from build123d import *

# Parameters (mm, degrees)
F2_ANGLE_BACK   = 15
F2_ANGLE        = 30
F2_COPIES_COUNT = 7


# Not quite as in the source:
# - a pattern or mirror of a feature is missing from the dataset's text; its kind, count and spacing are read off the source's solid


with BuildPart() as f1:
    # F0 (on Right) → F1 (revolve)
    with BuildSketch(Plane.YZ):
        Polygon((9.3, 4.0896662887), (9.3, 0), (12.9161745474, 0), (12.0366714414, 0.9946627731), (11.620462189, 0.6266412283), (9.8856947209, 2.5885542775), (10.3019039734, 2.9565758223), align=None)
        Polygon((11.620462189, 0.6266412283), (12.0366714414, 0.9946627731), (10.3019039734, 2.9565758223), (9.8856947209, 2.5885542775), align=None)
    revolve(axis=Axis((0, 0, 2.1812447902), (0, 0, 1)))

    # F0 (on Right) → F2 (revolve, cut)
    with BuildSketch(Plane.YZ, mode=Mode.PRIVATE) as f2_sk:
        Polygon((11.620462189, 0.6266412283), (12.0366714414, 0.9946627731), (10.3019039734, 2.9565758223), (9.8856947209, 2.5885542775), align=None)
    f2 = revolve(f2_sk.sketch.rotate(Axis((0, 0, 2.1812447902), (0, 0, -1)), -F2_ANGLE_BACK), axis=Axis((0, 0, 2.1812447902), (0, 0, -1)), revolution_arc=F2_ANGLE, mode=Mode.SUBTRACT)

    # F2_copies: F2 ×7 about axis
    f2_copies_axis = Axis((0, 0, 0), (0, 0, 1))
    for i in range(1, F2_COPIES_COUNT):
        add(f2.rotate(f2_copies_axis, i * 360 / F2_COPIES_COUNT), mode=Mode.SUBTRACT)


solid = f1.part
Geometry check sheet. Reference: the model listing, model coordinates, mm. A direction names the side the tool comes from. Give positions to 0.01 mm unless a question says otherwise; leave off trailing zeros. Write each loop counter-clockwise with the first axis right and the second up, starting at its lowest first coordinate (ties: lowest second). Pieces come first, ordered by that corner, then holes.
1) Set-up check for faces 1 (the face through (-0.04, 10.77, 1.59)), 2 (the face through (-9.2, 7.29, 0.73)), 3 (the face through (-9.785, -2.271, 2.729)): record each of +Z, -Z, +X, -X, +Y, -Y from which the full face is reachable in a straight line by a thin tool's end or side.
Values follow:
face 1: none
face 2: +Z
face 3: -X
2) Go/stop test with flat-tipped pins: pin 1 Ø1 at (y, z) = (-8, 3.5) entering from +X; pin 2 Ø1 at (y, z) = (6.5, 2.5) entering from +X; pin 3 Ø1 at (x, z) = (-6, 3) entering from -Y. Record where each tip stops, or that it passes through.
Values follow:
pin 1: stops at x = 6.65
pin 2: stops at x = 8.25
pin 3: stops at y = -8.71
3) Cross-section at A-A (y = 0). Record the boundary of the cut face in (x, z).
Values follow:
outline: (-12.92, 0) - (-9.3, 0) - (-9.3, 4.09) - (-10.3, 2.96) - (-9.89, 2.59) - (-11.62, 0.63) - (-12.04, 0.99) - close; (9.3, 0) - (12.92, 0) - (12.04, 0.99) - (11.62, 0.63) - (9.89, 2.59) - (10.3, 2.96) - (9.3, 4.09) - close
4) Cross-section at C-C (z = 3.3). Record the boundary of the cut face in (x, y).
Values follow:
outline: circle Ø20 at (0, 0); hole circle Ø18.6 at (0, 0)
5) Thickness scan on line 1 (X direction, y = 0, z = 0.8); line 2 (Y direction, x = 0.5, z = 0.8); line 3 (X direction, y = -4, z = 3.85). Record the ranges inside material, lowest first.
Values follow:
line 1: x = -12.21 to -11.82, -11.47 to -9.3, 9.3 to 11.47, 11.82 to 12.21
line 2: y = -12.2 to -9.29, 9.29 to 11.46, 11.81 to 12.2
line 3: x = -8.63 to -8.4, 8.4 to 8.63
6) Release check for a two-part mould opening along X. For faces 4 (the face through (-5.055, -10.595, 0.731)), 5 (the face through (-3, 9, 0)), 6 (the face through (9.8, -2.2, 2.73)) record: released by +X, released by -X, zero draft, split by the parting line, or undercut.
Values follow:
face 4: undercut
face 5: zero draft
face 6: released by +X
